Source: CAD feature listing. Evaluate the final solid. Frame: model axes, mm. Face numbers are marked on the shaded views. Give positions to 0.01 mm unless a question says otherwise; leave off trailing zeros. Loops run counter-clockwise (first coordinate to the right, second up) from the corner with the lowest first, then second, coordinate; pieces in that order, holes last. Notation, with made-up numbers: (41.5, -15.5) -> (83.5, -15.5) arc R7 ccw to (83.5, -8.5) -> close; hole circle Ø2 at (18, -9). An arc over 180 degrees is marked (long way). Return JSON: item names as keys, results as strings. Group by question number.
(1) Ray query, line 1 (X direction, y = 5.5, z = -8); line 2 (Z direction, x = -10, y = 7); line 3 (X direction, y = 7.75, z = -9.5). Return the intervals inside material, ascending. Write a range as from..to.
(2) Draft query along X for the marked faces 1, 2, 3 and 4. Return one class per face: released by +X, released by -X, zero draft, split by the parting line, or undercut.
(3) Cut plane B-B on z = -8. Return loops of the section in (x, y), then the cut area to 3 significant figures.
(4) Cut plane A-A on x = -10. Return loops of the section in (y, z), then the cut area to 4 significant figures.
(5) Pin query (flat end, axial travel): pin 1 (4 mm diameter, centred on x = -10, z = -8, fed in from -Y); pin 2 (2 mm diameter, centred on x = -8.5, z = -7, fed in from -Y). Return the tip coordinate at first contact, or that it passes through.
(6) Cut plane D-D on z = -9.5. Return loops of the section in (x, y).
(7) Cut plane C-C on y = 8.5. Return loops of the section in (x, z), then the cut area to 3 significant figures.
```python
from build123d import *

# Parameters (mm, degrees)
BOSS_EXTRUDE3_DEPTH           = 20.5
BOSS_EXTRUDE3_DEPTH_BACK      = 20.5
CUT_EXTRUDE1_DEPTH            = 30.004310025
CUT_EXTRUDE1_DEPTH_BACK       = 30.004310025
SKETCH5_W                     = 12
SKETCH5_H                     = 11
SPLIT1_SURFACE_1_BACK         = 57.187
SPLIT1_SURFACE_1_DEPTH        = 114.374
SPLIT1_SURFACE_2_BACK         = 57.187
SPLIT1_SURFACE_2_DEPTH        = 114.374
M5_TAPPED_HOLE1_AT_2_COUNT    = 2
M5_TAPPED_HOLE1_AT_2_PITCH    = 20
SKETCH13_W                    = 2.65
SKETCH13_H                    = 8.5
M5_CLEARANCE_HOLE1_AT_2_COUNT = 2
M5_CLEARANCE_HOLE1_AT_2_PITCH = 20
SKETCH4_W                     = 1.65
SKETCH4_H                     = 25.5
SKETCH4_AT_POINT_2_W          = 1.65
SKETCH4_AT_POINT_2_H          = 25.5
SKETCH4_AT_POINT_3_W          = 1.65
SKETCH4_AT_POINT_3_H          = 25.5
SKETCH4_AT_POINT_4_W          = 1.65
SKETCH4_AT_POINT_4_H          = 25.5
CHAMFER1_SIZE                 = 2
CHAMFER2_SIZE                 = 1
CHAMFER2_SIZE2                = 1.732050808
FILLET1_R                     = 0.2


with BuildPart() as part:
    # Sketch3 → Boss-Extrude3 (new, two sides: drawn at the far end of the back side and taken through both)
    with BuildSketch(Plane(origin=(0, 0, 0), x_dir=(1, 0, 0), z_dir=(0, 1, 0)).offset(-BOSS_EXTRUDE3_DEPTH_BACK)):
        Polygon((10.5, -10), (10.5, 0), (12.5, 0), (12.5, 2), (15, 2), (15, 14), (-15, 14), (-15, 2), (-10.5, 2), (-10.5, 0), (-10.5, -10), align=None)
    extrude(amount=BOSS_EXTRUDE3_DEPTH + BOSS_EXTRUDE3_DEPTH_BACK)

    # Sketch5 → Cut-Extrude1 (cut, two sides: drawn at the far end of the back side and taken through both)
    with BuildSketch(Plane(origin=(0, 0, 0), x_dir=(0, 0, -1), z_dir=(1, 0, 0)).offset(-CUT_EXTRUDE1_DEPTH_BACK)):
        Polygon((2, 0.5), (4.5, 0.5), (4.5, 1), (11.5, 1), (11.5, 0.5), (14, 0.5), (14, -0.5), (11.5, -0.5), (11.5, -1), (4.5, -1), (4.5, -0.5), (2, -0.5), align=None)
        with Locations((8, 15)):
            Rectangle(SKETCH5_W, SKETCH5_H)
    extrude(amount=CUT_EXTRUDE1_DEPTH + CUT_EXTRUDE1_DEPTH_BACK, mode=Mode.SUBTRACT)


with BuildPart() as body_2:
    # Split1: the piece behind the surface
    add(part.part)
    # Split1 surface: a surface, the sketch's curves swept straight by 114.374 mm
    with BuildLine(Plane.ZY.offset(10.5).offset(-SPLIT1_SURFACE_1_BACK), mode=Mode.PRIVATE) as split1_surface_1_path:
        Line((-2, 20.5), (-2, -0.5))
    split1_surface_1 = Shell.extrude(split1_surface_1_path.wire(), (-1 * SPLIT1_SURFACE_1_DEPTH, 0 * SPLIT1_SURFACE_1_DEPTH, 0 * SPLIT1_SURFACE_1_DEPTH))
    split(bisect_by=split1_surface_1, keep=Keep.BOTTOM)

    # Sketch13 → M5 Clearance Hole1 (revolve, cut)
    with BuildSketch(Plane(origin=(-10, 9.5, -8), x_dir=(0, 0, 1), z_dir=(1, 0, 0))):
        with Locations((1.325, 4.25)):
            Rectangle(SKETCH13_W, SKETCH13_H)
    m5_clearance_hole1 = revolve(axis=Axis((-10, 15.85, -8), (0, -1, 0)), mode=Mode.SUBTRACT)

    # M5 Clearance Hole1 at 2: M5 Clearance Hole1 ×2
    with Locations(*[(i * M5_CLEARANCE_HOLE1_AT_2_PITCH, 0, 0) for i in range(1, M5_CLEARANCE_HOLE1_AT_2_COUNT)]):
        add(m5_clearance_hole1, mode=Mode.SUBTRACT)


with BuildPart() as part_1:
    add(part.part)

    # Split1: split by a surface, the side it looks to stays
    # Split1 surface: a surface, the sketch's curves swept straight by 114.374 mm
    with BuildLine(Plane.ZY.offset(10.5).offset(-SPLIT1_SURFACE_2_BACK), mode=Mode.PRIVATE) as split1_surface_2_path:
        Line((-2, 20.5), (-2, -0.5))
    split1_surface_2 = Shell.extrude(split1_surface_2_path.wire(), (-1 * SPLIT1_SURFACE_2_DEPTH, 0 * SPLIT1_SURFACE_2_DEPTH, 0 * SPLIT1_SURFACE_2_DEPTH))
    split(bisect_by=split1_surface_2, keep=Keep.TOP)

    # Sketch10 → M5 Tapped Hole1 (revolve, cut)
    with BuildSketch(Plane(origin=(-10, -1, -8), x_dir=(0, 0, 1), z_dir=(1, 0, 0))):
        Polygon((0, 0), (0, 15.2618073), (2.1, 14), (2.1, 0), align=None)
    m5_tapped_hole1 = revolve(axis=Axis((-10, 5.35, -8), (0, -1, 0)), mode=Mode.SUBTRACT)

    # M5 Tapped Hole1 at 2: M5 Tapped Hole1 ×2
    with Locations(*[(i * M5_TAPPED_HOLE1_AT_2_PITCH, 0, 0) for i in range(1, M5_TAPPED_HOLE1_AT_2_COUNT)]):
        add(m5_tapped_hole1, mode=Mode.SUBTRACT)

    # Sketch4 → M4 Tapped Hole1 (revolve, cut)
    with BuildSketch(Plane(origin=(10.5, 12.5, 5), x_dir=(0, 0, -1), z_dir=(0, 1, 0))):
        with Locations((0.825, 12.75)):
            Rectangle(SKETCH4_W, SKETCH4_H)
    revolve(axis=Axis((10.5, 12.5, 3.35), (0, 0, 1)), mode=Mode.SUBTRACT)

    # Sketch4 at point 2 (carried to point 2, square into its face) → M4 Tapped Hole1 at 2 (revolve, cut)
    with BuildSketch(Plane(origin=(10.5, -12.5, 5), x_dir=(1, 0, 0), z_dir=(0, 1, 0))):
        with Locations((0.825, 12.75)):
            Rectangle(SKETCH4_AT_POINT_2_W, SKETCH4_AT_POINT_2_H)
    revolve(axis=Axis((12.15, -12.5, 5), (-1, 0, 0)), mode=Mode.SUBTRACT)

    # Sketch4 at point 3 (carried to point 3, square into its face) → M4 Tapped Hole1 at 3 (revolve, cut)
    with BuildSketch(Plane(origin=(-10.5, 12.5, 5), x_dir=(-1, 0, 0), z_dir=(0, 1, 0))):
        with Locations((0.825, 12.75)):
            Rectangle(SKETCH4_AT_POINT_3_W, SKETCH4_AT_POINT_3_H)
    revolve(axis=Axis((-12.15, 12.5, 5), (1, 0, 0)), mode=Mode.SUBTRACT)

    # Sketch4 at point 4 (carried to point 4, square into its face) → M4 Tapped Hole1 at 4 (revolve, cut)
    with BuildSketch(Plane(origin=(-10.5, -12.5, 5), x_dir=(-1, 0, 0), z_dir=(0, 1, 0))):
        with Locations((0.825, 12.75)):
            Rectangle(SKETCH4_AT_POINT_4_W, SKETCH4_AT_POINT_4_H)
    revolve(axis=Axis((-12.15, -12.5, 5), (1, 0, 0)), mode=Mode.SUBTRACT)

    # Chamfer1
    chamfer1_edges = [part_1.edges().sort_by_distance(p)[0] for p in [
        (-10.5, -20.5, -2),
        (10.5, -20.5, -2),
        (10.5, 20.5, 7.5),
        (-10.5, 20.5, 0.675),
    ]]
    chamfer(chamfer1_edges, length=CHAMFER1_SIZE)

    # Chamfer2
    chamfer2_edges = [part_1.edges().sort_by_distance(p)[0] for p in [
        (0, -20.5, 10),
        (10.5, 0, 10),
        (-1, 20.5, 10),
        (-10.5, 1, 10),
        (-1, 20.5, 10),
        (9.5, 19.5, 10),
        (-9.5, -19.5, 10),
        (9.5, -19.5, 10),
    ]]
    chamfer2_side = [part_1.faces().sort_by_distance(p)[0] for p in [
        (-0.023001949, 0.046393762, 10),
    ]]
    chamfer(chamfer2_edges, length=CHAMFER2_SIZE, length2=CHAMFER2_SIZE2, reference=chamfer2_side[0])

    # Fillet1
    fillet1_edges = [part_1.edges().sort_by_distance(p)[0] for p in [
        (0, -0.5, -2),
    ]]
    fillet(fillet1_edges, radius=FILLET1_R)


solid = body_2.part
```
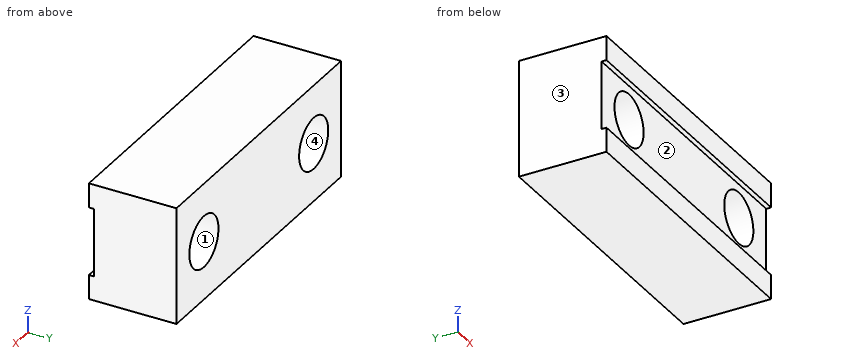
Answers:
{
 "1": {"line 1": "-15..-12.65, -7.35..7.35, 12.65..15", "line 2": "-14..-10.65, -5.35..-2", "line 3": "-15..-12.18, -7.82..7.82, 12.18..15"},
 "2": {"face 1": "undercut", "face 2": "zero draft", "face 3": "released by -X", "face 4": "undercut"},
 "3": {"outline": "(-15, 1) -> (-12.65, 1) -> (-12.65, 9.5) -> (-15, 9.5) -> close; (-7.35, 1) -> (7.35, 1) -> (7.35, 9.5) -> (-7.35, 9.5) -> close; (12.65, 1) -> (15, 1) -> (15, 9.5) -> (12.65, 9.5) -> close", "area": "165 mm²"},
 "4": {"outline": "(0.5, -14) -> (9.5, -14) -> (9.5, -10.65) -> (1, -10.65) -> (1, -11.5) -> (0.5, -11.5) -> close; (0.5, -4.5) -> (1, -4.5) -> (1, -5.35) -> (9.5, -5.35) -> (9.5, -2) -> (0.5, -2) -> close", "area": "59.45 mm²"},
 "5": {"pin 1": "through", "pin 2": "y = 1"},
 "6": {"outline": "(-15, 1) -> (-12.18, 1) -> (-12.18, 9.5) -> (-15, 9.5) -> close; (-7.82, 1) -> (7.82, 1) -> (7.82, 9.5) -> (-7.82, 9.5) -> close; (12.18, 1) -> (15, 1) -> (15, 9.5) -> (12.18, 9.5) -> close"},
 "7": {"outline": "(-15, -14) -> (15, -14) -> (15, -2) -> (-15, -2) -> close; hole circle Ø5.3 at (-10, -8); hole circle Ø5.3 at (10, -8)", "area": "316 mm²"}
}
